The listing builds one solid part. Answer for the finished solid, in the listing's coordinates (mm). Give positions to 0.01 mm unless a question says otherwise; leave off trailing zeros. Order: outer loops, then holes, each group sorted by start corner. A loop starts at its lowest first (then second) coordinate and runs counter-clockwise, first axis right, second up.
```python
from build123d import *

# Parameters (mm, degrees)
R_P_TITION_LIN_AIRE1_COUNT = 2
R_P_TITION_LIN_AIRE1_PITCH = 120
BOSS_EXTRU_1_REACH         = 132.767
BOSS_EXTRU_1_END_RADIUS    = 10
ESQUISSE2_R                = 2.5


with BuildPart() as part:
    # Esquisse1 → R_volution3 (revolve)
    with BuildSketch(Plane.XY):
        with BuildLine():
            Line((-10, 0), (10, 0))
            ThreePointArc((10, 0), (0, 10), (-10, 0))
        make_face()
    revolve(axis=Axis((-9.638277329, 0, 0), (1, 0, 0)))


with BuildPart() as r_p_tition_lin_aire1_1:
    # R_p_tition lin_aire1: pattern copy
    add(part.part.moved(Location(Vector(1, 0, 0) * (1 * R_P_TITION_LIN_AIRE1_PITCH))))


with BuildPart() as part_1:
    add(part.part)

    add(r_p_tition_lin_aire1_1.part)  # Boss.-Extru.1 merges R_p_tition lin_aire1_1
    # Boss.-Extru.1: up to this sphere (the profile starts outside it)
    boss_extru_1_end = Location((120, 0, 0)) * Sphere(BOSS_EXTRU_1_END_RADIUS, mode=Mode.PRIVATE)
    # Esquisse2 → Boss.-Extru.1 (add, up to the surface)
    with BuildSketch(Plane(origin=(0, 0, 0), x_dir=(0, 0, -1), z_dir=(1, 0, 0)), mode=Mode.PRIVATE) as boss_extru_1_sk1:
        with Locations(Location((0, 0, 0), (0, 0, 180))):
            Circle(ESQUISSE2_R)
    boss_extru_1_tool1 = extrude(boss_extru_1_sk1.sketch, amount=BOSS_EXTRU_1_REACH, mode=Mode.PRIVATE) - boss_extru_1_end
    add(boss_extru_1_tool1.solids().sort_by_distance((0, 0, 0))[0])


solid = part_1.part
```
1) Given P1, Ø10, axis at x = 38, z = 8, coming from the -Y side; P2, Ø12, axis at x = 33, y = -3, coming from the -Z side; P3, Ø10, axis at y = 0, z = 5.5, coming from the +X side; P4, Ø5, axis at y = 4, z = 1.5, coming from the -X side, each flat-ended and moving along its own axis, determine where each tip first touches the part or whether it passes through.
Geometry says:
P1: passes through
P2: stops at z = -2.5
P3: stops at x = 129.99
P4: stops at x = -9.84
2) Find section C-C (z = -4.25). Write down the section's boundary in (x, y), then the cut area to 3 significant figures.
Geometry says:
outline: circle Ø18.1 at (0, 0); circle Ø18.1 at (120, 0)
area: 515 mm2
3) Straight lines are drawn through the part: probe 1 along X at (y, z) = (-7, 2); probe 2 along X at (y, z) = (5.25, -4.25); probe 3 along Y at (x, z) = (84, -1). For each, find the intervals that lie inside material, in ascending order.
Geometry says:
probe 1: x = -6.86 to 6.86, 113.14 to 126.86
probe 2: x = -7.37 to 7.37, 112.63 to 127.37
probe 3: y = -2.29 to 2.29
4) Find section D-D (x = 76). Write down the section's boundary in (y, z), then the cut area to 3 significant figures.
Geometry says:
outline: circle Ø5 at (0, 0)
area: 19.6 mm2
5) Find section B-B (x = 120). Write down the section's boundary in (y, z).
Geometry says:
outline: circle Ø20 at (0, 0)
6) Find section A-A (y = -4). Write down the section's boundary in (x, z).
Geometry says:
outline: circle Ø18.33 at (0, 0); circle Ø18.33 at (120, 0)
